Design review of the part built by this model. Coordinates are the model's own, in mm. Coordinates: 2 decimals unless noted, no trailing zeros. Answer in a Markdown table with one row per item.
from build123d import *

# Parameters (mm, degrees)
SKETCH1_W           = 120
SKETCH1_H           = 60
BOSS_EXTRUDE1_DEPTH = 5
SKETCH1_6_R         = 1.5
CUT_EXTRUDE1_DEPTH  = 5
SKETCH1_7_R         = 3
CUT_EXTRUDE2_DEPTH  = 3
SKETCH1_12_R        = 3
CUT_EXTRUDE4_DEPTH  = 5
SKETCH1_13_R        = 3
SKETCH1_13_R_2      = 1.5
BOSS_EXTRUDE2_DEPTH = 2.5
FILLET1_R           = 5
SKETCH3_W           = 14
SKETCH3_H           = 14
CUT_EXTRUDE8_DEPTH  = 10


with BuildPart() as part:
    # Sketch1 → Boss-Extrude1 (new body)
    with BuildSketch(Plane.XY):
        with Locations((60, 30)):
            Rectangle(SKETCH1_W, SKETCH1_H)
    extrude(amount=BOSS_EXTRUDE1_DEPTH)

    # Sketch1_6 → Cut-Extrude1 (cut)
    with BuildSketch(Plane.XY):
        with Locations((4.5, 55.5)):
            Circle(SKETCH1_6_R)
        with Locations((4.5, 4.5)):
            Circle(SKETCH1_6_R)
        with Locations((115.5, 4.5)):
            Circle(SKETCH1_6_R)
        with Locations((115.5, 55.5)):
            Circle(SKETCH1_6_R)
    extrude(amount=CUT_EXTRUDE1_DEPTH, mode=Mode.SUBTRACT)

    # Sketch1_7 → Cut-Extrude2 (cut)
    with BuildSketch(Plane.XY):
        with Locations((4.5, 55.5)):
            Circle(SKETCH1_7_R)
        with Locations(Location((115.5, 55.5, 0), (0, 0, 180))):
            Circle(SKETCH1_7_R)
        with Locations(Location((4.5, 4.5, 0), (0, 0, 180))):
            Circle(SKETCH1_7_R)
        with Locations((115.5, 4.5)):
            Circle(SKETCH1_7_R)
    extrude(amount=CUT_EXTRUDE2_DEPTH, mode=Mode.SUBTRACT)

    # Sketch1_12 → Cut-Extrude4 (cut)
    with BuildSketch(Plane.XY):
        with Locations((37.019029611, 52.980970389)):
            Circle(SKETCH1_12_R)
        with Locations(Location((82.980970389, 52.980970389, 0), (0, 0, 180))):
            Circle(SKETCH1_12_R)
        with Locations(Location((37.019029611, 7.019029611, 0), (0, 0, 180))):
            Circle(SKETCH1_12_R)
        with Locations((82.980970389, 7.019029611)):
            Circle(SKETCH1_12_R)
    extrude(amount=CUT_EXTRUDE4_DEPTH, mode=Mode.SUBTRACT)

    # Sketch1_13 → Boss-Extrude2 (add)
    # profile 1 of 4: a face of its own
    with BuildSketch(Plane.XY):
        with Locations(Location((82.980970389, 52.980970389, 0), (0, 0, 180))):
            Circle(SKETCH1_13_R)
        with Locations((82.980970389, 52.980970389)):
            Circle(SKETCH1_13_R_2, mode=Mode.SUBTRACT)
    # profile 2 of 4: a face of its own
    with BuildSketch(Plane.XY):
        with Locations((82.980970389, 7.019029611)):
            Circle(SKETCH1_13_R)
        with Locations((82.980970389, 7.019029611)):
            Circle(SKETCH1_13_R_2, mode=Mode.SUBTRACT)
    # profile 3 of 4: a face of its own
    with BuildSketch(Plane.XY):
        with Locations((37.019029611, 52.980970389)):
            Circle(SKETCH1_13_R)
        with Locations((37.019029611, 52.980970389)):
            Circle(SKETCH1_13_R_2, mode=Mode.SUBTRACT)
    # profile 4 of 4: a face of its own
    with BuildSketch(Plane.XY):
        with Locations(Location((37.019029611, 7.019029611, 0), (0, 0, 180))):
            Circle(SKETCH1_13_R)
        with Locations((37.019029611, 7.019029611)):
            Circle(SKETCH1_13_R_2, mode=Mode.SUBTRACT)
    extrude(amount=BOSS_EXTRUDE2_DEPTH)

    # Fillet1
    fillet1_edges = [part.edges().sort_by_distance(p)[0] for p in [
        (0, 0, 2.5),
        (0, 60, 2.5),
        (120, 60, 2.5),
        (120, 0, 2.5),
    ]]
    fillet(fillet1_edges, radius=FILLET1_R)

    # Sketch3 → Cut-Extrude8 (cut)
    with BuildSketch(Plane.XY):
        with Locations((60, 18)):
            Rectangle(SKETCH3_W, SKETCH3_H)
        with Locations((60, 42)):
            Rectangle(SKETCH3_W, SKETCH3_H)
    extrude(amount=CUT_EXTRUDE8_DEPTH, mode=Mode.SUBTRACT)


solid = part.part
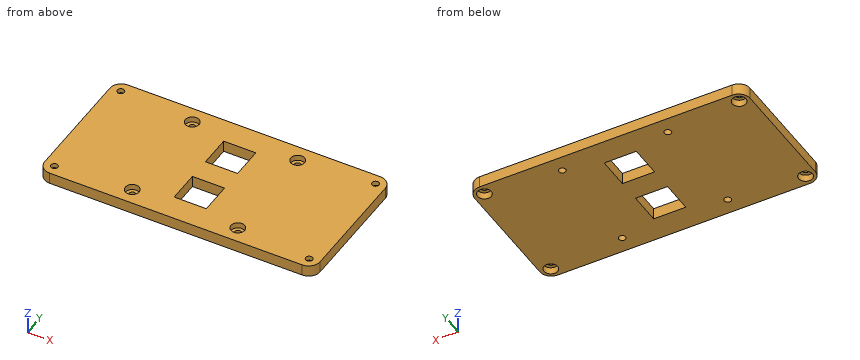
(1) Add section A-A, the plane z = 3.8. Give the number of separate pieces and of enclosed holes in the cut face, and give its area (3 significant figures).
Return value:
| item | result |
|---|---|
| separate pieces | 1 |
| enclosed holes | 10 |
| area | 6,650 mm2 |
(2) For line 1 along Y through (x, z) = (115.5, 3.5); line 2 along Y through (x, z) = (57, 3.5); line 3 along X through (y, z) = (37.5, 4.6), list the stretches that pass through material, from the lowest coordinate up. Write a range as from..to.
Return value:
| item | result |
|---|---|
| line 1 | y = 0.03..3, 6..54, 57..59.97 |
| line 2 | y = 0..11, 25..35, 49..60 |
| line 3 | x = 0..53, 67..120 |
(3) Insertion check: pin 1 Ø5.5 at (x, y) = (4.5, 55.5) entering from -Z; pin 2 Ø3.5 at (x, y) = (82.98, 52.98) entering from +Z. Each pin has a flat end and moves straight along its axis. Give the tip position at first contact, or say it passes through.
Return value:
| item | result |
|---|---|
| pin 1 | stops at z = 3 |
| pin 2 | stops at z = 2.5 |
